Autodesk Inventor part; units mm, degrees
ref_plane "YZ Plane" through (0, 0, 0) normal (1, 0, 0) x (0, 1, 0)
ref_plane "XZ Plane" through (0, 0, 0) normal (0, 1, 0) x (-1, 0, 0)
ref_plane "XY Plane" through (0, 0, 0) normal (0, 0, 1) x (1, 0, 0)
sketch "スケッチ1" plane through (0, 0, 0) normal (0, 0, 1) x (1, 0, 0)
  line L0 (-12.5, 5) -> (12.5, 5)
  line L1 (12.5, 5) -> (12.5, -5)
  line L2 (12.5, -5) -> (-12.5, -5)
  line L3 (-12.5, -5) -> (-12.5, 5)
  line L4 (-12.5, 5) -> (12.5, -5) construction
  line L5 (12.5, 5) -> (-12.5, -5) construction
  point P0 (0, 0)
  dimension "d0" = 25
  dimension "d1" = 10
extrude "押し出し1" add sketch "スケッチ1" along normal blind 1
sketch "スケッチ3" plane through (0, 0, 1) normal (0, 0, 1) x (1, 0, 0)
  line L0 (-12.5, 5) -> (12.5, 5)
  line L1 (12.5, 5) -> (12.5, 6)
  line L2 (12.5, 6) -> (-12.5, 6)
  line L3 (-12.5, 6) -> (-12.5, 5)
  point P0 (0, 0)
  dimension "d15" = 25
  dimension "d16" = 1
extrude "押し出し2" add sketch "スケッチ3" against normal blind 11
sketch "スケッチ7" plane through (0, 0, 0) normal (0, 0, -1) x (-1, 0, 0)
  line L0 (12.5, -5) -> (-12.5, -5)
  line L1 (-12.5, -5) -> (-12.5, 5)
  line L2 (-12.5, 5) -> (12.5, 5)
  line L3 (12.5, 5) -> (12.5, -5)
  point P0 (0, 0)
extrude "押し出し4" add sketch "スケッチ7" along normal blind 0.5
sketch "スケッチ8" plane through (-12.5, 5, -10) normal (0, -1, 0) x (1, 0, 0)
  line L0 (0, 0) -> (25, 0)
  line L1 (25, 0) -> (25, 9.5)
  line L2 (25, 9.5) -> (0, 9.5)
  line L3 (0, 9.5) -> (0, 0)
  point P0 (12.5, 10)
extrude "押し出し5" add sketch "スケッチ8" along normal blind 0.5
sketch "スケッチ9" plane through (0, 0, 1) normal (0, 0, 1) x (1, 0, 0)
  line L0 (-12.5, 4.5) -> (12.5, 4.5)
  line L1 (12.5, -5) -> (12.5, 6)
  line L2 (-12.5, 6) -> (-12.5, -5)
  point P0 (0, 0)
  point P1 (7.5, 0)
  point P2 (-7.5, 0)
  dimension "d38" = 4.5
  dimension "d39" = 5
  dimension "d40" = 5
  dimension "d41" = 4.5
hole "穴3" at (7.5, 0, 1) at (-7.5, 0, 1) direction (0, 0, -1) diameter 3.2 depth 8 tip angle 118
sketch "スケッチ10" plane through (-12.5, 6, 1) normal (0, 1, 0) x (1, 0, 0)
  line L0 (0, 11) -> (25, 11)
  line L1 (25, 0) -> (25, 11)
  point P0 (12.5, 1)
  point P1 (4.5, 7)
  point P2 (20.5, 7)
  dimension "d49" = 4
  dimension "d50" = 4.5
  dimension "d51" = 4
  dimension "d52" = 16
hole "穴4" at (-8, 6, -6) at (8, 6, -6) direction (0, -1, 0) diameter 2.2 depth 8 tip angle 118
properties part number "Servo catch" material "アルミニウム 1100-H14"
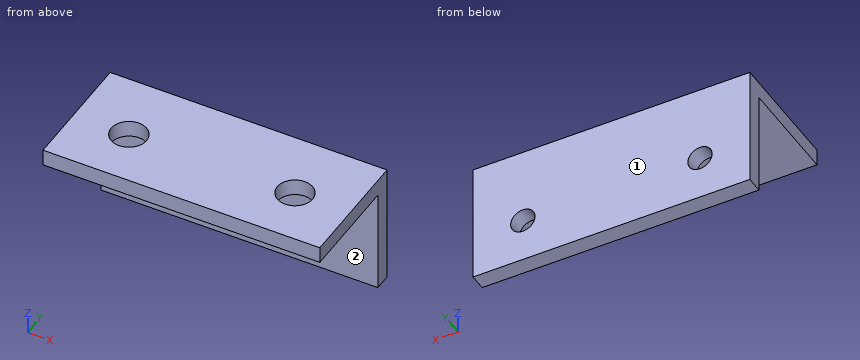
Read the model definition and answer for the solid it produces. Units are mm, in the model's axes. Face numbers are marked on the shaded views. A direction names the side the tool comes from. Give positions to 0.01 mm unless a question says otherwise; leave off trailing zeros. Order: outer loops, then holes, each group sorted by start corner. A loop starts at its lowest first (then second) coordinate and runs counter-clockwise, first axis right, second up.
(1) Find section C-C (x = -7.5). Give the vertices of the cut face in (y, z), plus the area to 3 significant figures.
(2) Find section D-D (x = 9.5). Give the vertices of the cut face in (y, z).
(3) Find section A-A (y = 0). Give the vertices of the cut face in (x, z), plus the area to 3 significant figures.
(4) Given pin 1 (6 mm diameter, centred on x = -0.5, y = -3.5, fed in from -Z); pin 2 (3 mm diameter, centred on x = -8, z = -6, fed in from -Y), each flat-ended and moving along its own axis, determine where each tip first touches the part or whether it passes through.
(5) Straight lines are drawn through the part: L1, parallel to X at y = 0, z = 0.7; L2, parallel to X at y = 5.25, z = -6; L3, parallel to Z at x = 8, y = 5.2. For each, find the intervals that lie inside material, in ascending order.
(6) Find section B-B (z = -6). Give the vertices of the cut face in (x, y), plus the area to 3 significant figures.
(7) For the marked faces 1 and 2, determine the directions among +Z, -Z, +X, -X, +Y, -Y from which every point of the face is accessible in a straight line to the end or side of a thin tool.
Result sheet:
1. outline: (-5, -0.5) - (-1.6, -0.5) - (-1.6, 1) - (-5, 1) - close; (1.6, -0.5) - (4.5, -0.5) - (4.5, -5.02) - (6, -5.02) - (6, 1) - (1.6, 1) - close; (4.5, -10) - (6, -10) - (6, -6.98) - (4.5, -6.98) - close
1. area: 23.0 mm2
2. outline: (-5, -0.5) - (4.5, -0.5) - (4.5, -10) - (6, -10) - (6, 1) - (-5, 1) - close
3. outline: (-12.5, -0.5) - (-9.1, -0.5) - (-9.1, 1) - (-12.5, 1) - close; (-5.9, -0.5) - (5.9, -0.5) - (5.9, 1) - (-5.9, 1) - close; (9.1, -0.5) - (12.5, -0.5) - (12.5, 1) - (9.1, 1) - close
3. area: 27.9 mm2
4. pin 1: stops at z = -0.5
4. pin 2: stops at y = 4.5
5. L1: x = -12.5 to -9.1, -5.9 to 5.9, 9.1 to 12.5
5. L2: x = -12.5 to -9.1, -6.9 to 6.9, 9.1 to 12.5
5. L3: z = -10 to -7.1, -4.9 to 1
6. outline: (-12.5, 4.5) - (-9.1, 4.5) - (-9.1, 6) - (-12.5, 6) - close; (-6.9, 4.5) - (6.9, 4.5) - (6.9, 6) - (-6.9, 6) - close; (9.1, 4.5) - (12.5, 4.5) - (12.5, 6) - (9.1, 6) - close
6. area: 30.9 mm2
7. face 1: +Z, -Z, +X, -X, +Y
7. face 2: -Z, +X, -X, -Y
